Geometry check sheet. Reference: the model listing, model coordinates, mm. Face numbers are marked on the shaded views. A direction names the side the tool comes from. Coordinates: 2 decimals unless noted, no trailing zeros. Order: outer loops, then holes, each group sorted by start corner. A loop starts at its lowest first (then second) coordinate and runs counter-clockwise, first axis right, second up. Notation, with made-up numbers: (45.25, -19) - (89.25, -19) arc R14 ccw to (89.25, 4) - close; hole circle Ø9 at (23, -20). An arc over 180 degrees is marked (long way). Return JSON: item names as keys, results as strings. Group by question number.
Item 1: Section check A-A on z = -5. Enter the section's corners in (x, y), then the cut area to 3 significant figures.
Item 2: Scan lines: probe 1 along X at (y, z) = (3.75, -1.5); probe 2 along X at (y, z) = (6.5, -32); probe 3 along Y at (x, z) = (-45, 1.45). Record each from-to range of solid material in increasing order.
Item 3: Gauge pin test, flat ends, axial feed: pin 1 (5 mm diameter, centred on y = 4.5, z = -30.5, fed in from -X); pin 2 (5 mm diameter, centred on x = -25.5, y = 7.5, fed in from -Z); pin 3 (5 mm diameter, centred on y = 6.5, z = -31, fed in from +X); pin 4 (4 mm diameter, centred on x = -25, y = 7.5, fed in from +Z). Record the tip position at first contact, or that the pin passes through.
Item 4: Draft check along X on the marked faces 4, 5 and 6. Enter one of: pulls with the +X half, pulls with the -X half, needs draft (parallel to the pull), parting line crosses it, or undercut.
Item 5: Tool access check on the marked faces 1, 2 and 3. Record the directions out of +Z, -Z, +X, -X, +Y, -Y that give a thin tool (end or side, any length) a straight path to the whole face; none if there is none.
Item 6: Section check B-B on x = -60.5. Enter the section's corners in (y, z), then the cut area to 3 significant figures.
Item 7: Section check C-C on y = 3.5. Enter the section's corners in (x, z) (3 decimals), then the cut area to 3 significant figures.
Item 8: Section check D-D on x = -35.05. Give the number of separate pieces and of enclosed holes in the cut face, then the cut area to 3 significant figures.
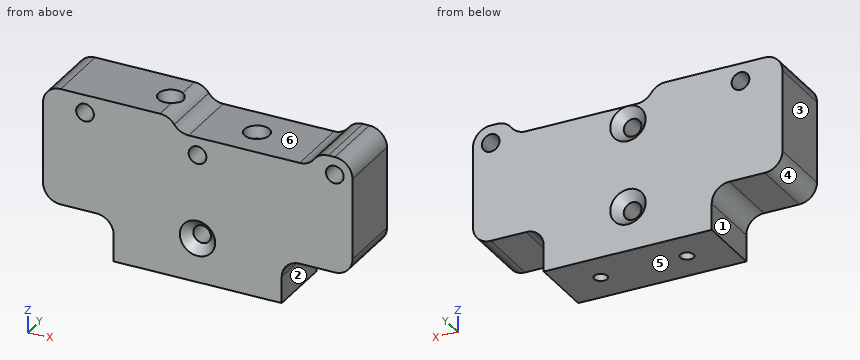
from build123d import *

# Parameters (mm, degrees)
SKETCH1_W           = 70
SKETCH1_H           = 34
SKETCH1_R           = 2
BOSS_EXTRUDE1_DEPTH = 15
SKETCH6_W           = 70
SKETCH6_H           = 15
BOSS_EXTRUDE2_DEPTH = 5
SKETCH3_R           = 2
CUT_EXTRUDE2_DEPTH  = 15
SKETCH8_W           = 6
SKETCH8_H           = 5
CUT_EXTRUDE3_DEPTH  = 15
SKETCH9_W           = 12
SKETCH9_H           = 6
CUT_EXTRUDE4_DEPTH  = 15
SKETCH10_W          = 16
SKETCH10_H          = 10
CUT_EXTRUDE5_DEPTH  = 17
SKETCH12_R          = 1.5
CUT_EXTRUDE6_DEPTH  = 41
SKETCH13_W          = 27.5
SKETCH13_H          = 6
CUT_EXTRUDE7_DEPTH  = 20
SKETCH14_W          = 13.5
SKETCH14_H          = 2.67
SKETCH14_W_2        = 29
CUT_EXTRUDE8_DEPTH  = 17
FILLET2_R           = 4
SKETCH16_W          = 5.5
SKETCH16_H          = 3.33
CUT_EXTRUDE10_DEPTH = 18
FILLET4_R           = 4
FILLET5_R           = 4
SKETCH17_R          = 2.85
CUT_EXTRUDE11_DEPTH = 3
SKETCH18_R          = 2.8
CUT_EXTRUDE12_DEPTH = 3
CHAMFER1_SIZE       = 2


# Some blends are built 0.0001 mm under size
with BuildPart() as part:
    # Sketch1 → Boss-Extrude1 (new body)
    with BuildSketch(Plane(origin=(0, 0, 0), x_dir=(1, 0, 0), z_dir=(0, 1, 0))):
        with Locations((-35, 17)):
            Rectangle(SKETCH1_W, SKETCH1_H)
        with Locations(Location((-35.05, 24, 0), (0, 0, 270))):
            Circle(SKETCH1_R, mode=Mode.SUBTRACT)
        with Locations(Location((-35.05, 5, 0), (0, 0, 270))):
            Circle(SKETCH1_R, mode=Mode.SUBTRACT)
    extrude(amount=BOSS_EXTRUDE1_DEPTH)

    # Sketch6 → Boss-Extrude2 (add)
    with BuildSketch(Plane.XY):
        with Locations((-35, 7.5)):
            Rectangle(SKETCH6_W, SKETCH6_H)
    extrude(amount=BOSS_EXTRUDE2_DEPTH)

    # Sketch3 → Cut-Extrude2 (cut)
    with BuildSketch(Plane(origin=(0, 15, 0), x_dir=(1, 0, 0), z_dir=(0, 1, 0))):
        with Locations(Location((-4, 1.67, 0), (0, 0, 270))):
            Circle(SKETCH3_R)
        with Locations(Location((-60.5, 1.67, 0), (0, 0, 270))):
            Circle(SKETCH3_R)
    extrude(amount=-CUT_EXTRUDE2_DEPTH, mode=Mode.SUBTRACT)

    # Sketch8 → Cut-Extrude3 (cut)
    with BuildSketch(Plane(origin=(0, 15, 0), x_dir=(1, 0, 0), z_dir=(0, 1, 0))):
        with Locations((-16.5, -2.5)):
            Rectangle(SKETCH8_W, SKETCH8_H)
    extrude(amount=-CUT_EXTRUDE3_DEPTH, mode=Mode.SUBTRACT)

    # Sketch9 → Cut-Extrude4 (cut)
    with BuildSketch(Plane(origin=(0, 15, 0), x_dir=(1, 0, 0), z_dir=(0, 1, 0))):
        with Locations((-35, -2)):
            Rectangle(SKETCH9_W, SKETCH9_H)
    extrude(amount=-CUT_EXTRUDE4_DEPTH, mode=Mode.SUBTRACT)

    # Sketch10 → Cut-Extrude5 (cut)
    with BuildSketch(Plane.XZ):
        with Locations((-8, -29)):
            Rectangle(SKETCH10_W, SKETCH10_H)
        with Locations((-62, -29)):
            Rectangle(SKETCH10_W, SKETCH10_H)
    extrude(amount=-CUT_EXTRUDE5_DEPTH, mode=Mode.SUBTRACT)

    # Sketch12 → Cut-Extrude6 (cut)
    with BuildSketch(Plane.XY.offset(5)):
        with Locations((-44.5, 7.5)):
            Circle(SKETCH12_R)
        with Locations((-25, 7.499999999)):
            Circle(SKETCH12_R)
    extrude(amount=-CUT_EXTRUDE6_DEPTH, mode=Mode.SUBTRACT)

    # Sketch13 → Cut-Extrude7 (cut)
    with BuildSketch(Plane(origin=(0, 15, 0), x_dir=(1, 0, 0), z_dir=(0, 1, 0))):
        with Locations((-27.25, -2)):
            Rectangle(SKETCH13_W, SKETCH13_H)
    extrude(amount=-CUT_EXTRUDE7_DEPTH, mode=Mode.SUBTRACT)

    # Sketch14 → Cut-Extrude8 (cut)
    with BuildSketch(Plane(origin=(0, 0, 0), x_dir=(-1, 0, 0), z_dir=(0, -1, 0))):
        with Locations((6.75, -3.665)):
            Rectangle(SKETCH14_W, SKETCH14_H)
        with Locations((55.5, -3.665)):
            Rectangle(SKETCH14_W_2, SKETCH14_H)
    extrude(amount=-CUT_EXTRUDE8_DEPTH, mode=Mode.SUBTRACT)

    # Fillet2
    fillet2_edges = [part.edges().sort_by_distance(p)[0] for p in [
        (0, 7.5, 2.33),
        (-70, 7.5, 2.33),
        (-70, 7.5, -24),
        (0, 7.5, -24),
    ]]
    fillet(fillet2_edges, radius=FILLET2_R)

    # Sketch16 → Cut-Extrude10 (cut)
    with BuildSketch(Plane.XZ):
        with Locations((-10.75, 0.665)):
            Rectangle(SKETCH16_W, SKETCH16_H)
    extrude(amount=-CUT_EXTRUDE10_DEPTH, mode=Mode.SUBTRACT)

    # Fillet4
    # the kernel refuses this fillet: 4 mm, written as the material it adds along each edge
    with BuildSketch(Plane(origin=(-16, 0, -24), x_dir=(1, 0, 0), z_dir=(0, 1, 0)), Plane(origin=(-54, 0, -24), x_dir=(0, 0, -1), z_dir=(0, 1, 0))) as fillet4_piece_1:
        with BuildLine():
            CenterArc((FILLET4_R, FILLET4_R), FILLET4_R, 180, 90)
            Line((0, FILLET4_R), (-FILLET4_R * 0.02, FILLET4_R))
            Line((-FILLET4_R * 0.02, FILLET4_R), (-FILLET4_R * 0.02, -FILLET4_R * 0.02))
            Line((-FILLET4_R * 0.02, -FILLET4_R * 0.02), (FILLET4_R, -FILLET4_R * 0.02))
            Line((FILLET4_R, -FILLET4_R * 0.02), (FILLET4_R, 0))
        make_face()
    extrude(amount=15)
    with BuildSketch(Plane(origin=(-41, 15, -1), x_dir=(0, 0, 1), z_dir=(0, -1, 0))) as fillet4_piece_2:
        with BuildLine():
            CenterArc((4, -3.943488304), FILLET4_R, 99.642495459, 80.357504541)
            Line((0, -3.943488304), (-0.08, -3.943488304))
            Line((-0.08, -3.943488304), (-0.08, 0))
            Line((-0.08, 0), (0, 0.08))
            ThreePointArc((0, 0.08), (1.665, 0.08), (3.3166, 0.078869766))
            Line((3.3166, 0.078869766), (3.33, 0))
        make_face()
    extrude(amount=15)
    with BuildSketch(Plane(origin=(-8, 0, -1), x_dir=(-1.0, 0, -8.691057696161095e-11), z_dir=(0, 1, 0))) as fillet4_piece_3:
        with BuildLine():
            CenterArc((3.943488303, 4), FILLET4_R, 189.642495464, 80.357504541)
            Line((0, 3.33), (-0.078869766, 3.3166))
            ThreePointArc((-0.078869766, 3.3166), (-0.08, 1.665), (-0.08, 0))
            Line((-0.08, 0), (0, -0.08))
            Line((0, -0.08), (3.943488304, -0.08))
            Line((3.943488304, -0.08), (3.943488304, 0))
        make_face()
    extrude(amount=15)

    # Fillet5
    # the kernel refuses this fillet: 4 mm, written as the material it takes off along each edge
    with BuildSketch(Plane(origin=(-41, -6.379948368, 2.33), x_dir=(0.3855616700587326, 0, -0.922682067985241), z_dir=(0, 1, 0))) as fillet5_piece_1:
        with BuildLine():
            CenterArc((2.706782853, 3.896912262), FILLET5_R, 202.67861385, 54.285267758)
            Line((-0.983945419, 2.354665582), (0, 0))
            ThreePointArc((0, 0), (0.902260951, 0.103087738), (1.804521902, 0))
        make_face()
    extrude(amount=27.759896736, mode=Mode.SUBTRACT)
    with BuildSketch(Plane(origin=(-8, -6.379948368, 2.33), x_dir=(-0.38556167005872005, 0, -0.9226820679852463), z_dir=(0, 1, 0))) as fillet5_piece_2:
        with BuildLine():
            CenterArc((2.706782853, -3.896912262), FILLET5_R, 103.036118392, 54.285267758)
            Line((-0.983945419, -2.354665582), (0, 0))
            ThreePointArc((0, 0), (0.902260951, -0.103087738), (1.804521902, 0))
        make_face()
    extrude(amount=27.759896736, mode=Mode.SUBTRACT)

    # Sketch17 → Cut-Extrude11 (cut)
    with BuildSketch(Plane.XY.offset(-1)):
        with Locations((-25.499999999, 7.499999999)):
            Circle(SKETCH17_R)
    extrude(amount=-CUT_EXTRUDE11_DEPTH, mode=Mode.SUBTRACT)

    # Sketch18 → Cut-Extrude12 (cut)
    with BuildSketch(Plane.XY.offset(2.33)):
        with Locations((-45, 7.5)):
            Circle(SKETCH18_R)
    extrude(amount=-CUT_EXTRUDE12_DEPTH, mode=Mode.SUBTRACT)

    # Chamfer1
    chamfer1_edges = [part.edges().sort_by_distance(p)[0] for p in [
        (-35.05, 0, -26),
        (-35.05, 15, -26),
        (-35.05, 15, -7),
    ]]
    chamfer(chamfer1_edges, length=CHAMFER1_SIZE - 0.0001)  # a hair under: the kernel refuses the full size


solid = part.part
Computed:
{
 "1": {"outline": "(-70, 0) - (-37.05, 0) - (-37.05, 13) - (-39.05, 15) - (-70, 15) - close; (-33.05, 0) - (0, 0) - (0, 15) - (-31.05, 15) - (-33.05, 13) - close; hole circle Ø3 at (-44.5, 7.5); hole circle Ø3 at (-25, 7.5)", "area": "972 mm²"},
 "2": {"probe 1": "x = -70 to -62.49, -58.51 to -5.99, -2.01 to 0", "probe 2": "x = -54 to -45.62, -43.38 to -26.12, -23.88 to -16", "probe 3": "y = 0 to 4.7, 10.3 to 15"},
 "3": {"pin 1": "stops at x = -54", "pin 2": "stops at z = -34", "pin 3": "stops at x = -16", "pin 4": "stops at z = -4"},
 "4": {"face 4": "pulls with the -X half", "face 5": "needs draft", "face 6": "undercut"},
 "5": {"face 1": "-Z, -X, +Y, -Y", "face 2": "-Z, +X, +Y, -Y", "face 3": "+Z, -Z, -X, +Y, -Y"},
 "6": {"outline": "(0, -24) - (15, -24) - (15, -3.67) - (0, -3.67) - close; (0, 0.33) - (15, 0.33) - (15, 2.33) - (0, 2.33) - close", "area": "335 mm²"},
 "7": {"outline": "(-70, -20) arc R4 ccw to (-66, -24) - (-58, -24) arc R4 cw to (-54, -28) - (-54, -34) - (-16, -34) - (-16, -28) arc R4 cw to (-12, -24) - (-4, -24) arc R4 ccw to (0, -20) - (0, -1.67) arc R4 ccw to (-4, 2.33) - (-5.448, 2.33) arc R4 ccw to (-8.696, 0.665) arc R4 cw to (-11.943, -1) - (-37.057, -1) arc R4 cw to (-40.304, 0.665) arc R4 ccw to (-43.552, 2.33) - (-66, 2.33) arc R4 ccw to (-70, -1.67) - close; hole circle Ø4 at (-60.5, -1.67); hole circle Ø4 at (-35.05, -24); hole circle Ø4 at (-35.05, -5); hole circle Ø4 at (-4, -1.67)", "area": "2,060 mm²"},
 "8": {"separate pieces": "3", "enclosed holes": "0", "area": "363 mm²"}
}
